```python
from build123d import *
from build123d import SkipClean  # not in build123d's __all__

# Parameters (mm, degrees)
F0_R     = 0.4
F1_DEPTH = 1.4
F2_DEPTH = 2.3
F3_DEPTH = 0.5


with BuildPart() as f1:
    # F0 (on Top) → F1 (new body)
    with BuildSketch(Plane.XY):
        with BuildLine():
            ThreePointArc((-2.7, 2.1476731595), (-1.1374313166, -3.2571076126), (3.45, 0))
            ThreePointArc((3.45, 0), (3.2571076126, 1.1374313166), (2.7, 2.1476731595))
            Line((2.7, 2.1476731595), (1.0139649895, 2.1476731595))
            ThreePointArc((1.0139649895, 2.1476731595), (2.0060897101, 1.2713099838), (2.375, 0))
            ThreePointArc((2.375, 0), (-1.2713099838, -2.0060897101), (-1.0139649895, 2.1476731595))
            Line((-1.0139649895, 2.1476731595), (-2.7, 2.1476731595))
        make_face()
        with BuildLine():
            Line((1.0139649895, 2.1476731595), (2.7, 2.1476731595))
            ThreePointArc((2.7, 2.1476731595), (0, 3.45), (-2.7, 2.1476731595))
            Line((-2.7, 2.1476731595), (-1.0139649895, 2.1476731595))
            ThreePointArc((-1.0139649895, 2.1476731595), (0, 2.375), (1.0139649895, 2.1476731595))
        make_face()
        with BuildLine():
            ThreePointArc((-2.7, 2.1476731595), (0, 3.45), (2.7, 2.1476731595))
            Line((2.7, 2.1476731595), (2.0471920173, 14.6072606371))
            ThreePointArc((2.0471920173, 14.6072606371), (2.0492978841, 14.553648693), (2.05, 14.5))
            ThreePointArc((2.05, 14.5), (-0.053648693, 12.4507021159), (-2.0471920173, 14.6072606371))
            Line((-2.0471920173, 14.6072606371), (-2.7, 2.1476731595))
        make_face()
        with BuildLine():
            ThreePointArc((2.05, 14.5), (2.0492978841, 14.553648693), (2.0471920173, 14.6072606371))
            ThreePointArc((2.0471920173, 14.6072606371), (0, 16.55), (-2.0471920173, 14.6072606371))
            ThreePointArc((-2.0471920173, 14.6072606371), (-0.053648693, 12.4507021159), (2.05, 14.5))
        make_face()
        with Locations((0, 14.5)):
            Circle(F0_R, mode=Mode.SUBTRACT)
    extrude(amount=F1_DEPTH)

    # F0 (on Top) → F2 (join)
    with BuildSketch(Plane.XY):
        with BuildLine():
            Line((1.0139649895, 2.1476731595), (2.7, 2.1476731595))
            ThreePointArc((2.7, 2.1476731595), (0, 3.45), (-2.7, 2.1476731595))
            Line((-2.7, 2.1476731595), (-1.0139649895, 2.1476731595))
            ThreePointArc((-1.0139649895, 2.1476731595), (0, 2.375), (1.0139649895, 2.1476731595))
        make_face()
        with BuildLine():
            ThreePointArc((-2.7, 2.1476731595), (-1.1374313166, -3.2571076126), (3.45, 0))
            ThreePointArc((3.45, 0), (3.2571076126, 1.1374313166), (2.7, 2.1476731595))
            Line((2.7, 2.1476731595), (1.0139649895, 2.1476731595))
            ThreePointArc((1.0139649895, 2.1476731595), (2.0060897101, 1.2713099838), (2.375, 0))
            ThreePointArc((2.375, 0), (-1.2713099838, -2.0060897101), (-1.0139649895, 2.1476731595))
            Line((-1.0139649895, 2.1476731595), (-2.7, 2.1476731595))
        make_face()
    with SkipClean():  # cleaning this boolean's faces spoils the solid; the shape is the same uncleaned
        extrude(amount=-F2_DEPTH)

    # F0 (on Top) → F3 (join)
    with BuildSketch(Plane.XY):
        with BuildLine():
            Line((0, 2.1476731595), (1.0139649895, 2.1476731595))
            ThreePointArc((1.0139649895, 2.1476731595), (0, 2.375), (-1.0139649895, 2.1476731595))
            Line((-1.0139649895, 2.1476731595), (0, 2.1476731595))
        make_face()
        with BuildLine():
            ThreePointArc((2.375, 0), (2.0060897101, 1.2713099838), (1.0139649895, 2.1476731595))
            Line((1.0139649895, 2.1476731595), (0, 2.1476731595))
            Line((0, 2.1476731595), (-1.0139649895, 2.1476731595))
            ThreePointArc((-1.0139649895, 2.1476731595), (-1.2713099838, -2.0060897101), (2.375, 0))
        make_face()
        with BuildLine():
            ThreePointArc((1.175, 0), (-0.8308504679, -0.8308504679), (0, 1.175))
            ThreePointArc((0, 1.175), (0.8308504679, 0.8308504679), (1.175, 0))
        make_face(mode=Mode.SUBTRACT)
    extrude(amount=F3_DEPTH)


solid = f1.part
```
Can you work these out from the model? Positions are in its coordinate system, mm. A direction names the side the tool comes from. Give positions to 0.01 mm unless a question says otherwise; leave off trailing zeros. Order: outer loops, then holes, each group sorted by start corner. A loop starts at its lowest first (then second) coordinate and runs counter-clockwise, first axis right, second up. Notation, with made-up numbers: (88.5, -26) - (118.5, -26) arc R29 ccw to (118.5, 2) - close; hole circle Ø4 at (-22.5, 9.25). An arc over 180 degrees is marked (long way). Use a Markdown table: item, result. Add a question column.
Q1. Please list where these lines run through material, in increasing order: line 1 along X through (y, z) = (0, 0.4) (3 decimals); line 2 along Z through (x, y) = (-1.5, 4.5); line 3 along Y through (x, z) = (1, 0.9).
Q2. If we mould it in two halves opening along X, with no side actions, what happens to faces 3 (the flat face through (-2.37, 8.46, 0.69)), 4 (the flat face through (0, 9, 0)), 5 (the flat face through (-1, 1, 0.5)), 6 (the flat face through (2.38, 8.29, 0.69))? For each: released by +X, released by -X, zero draft, split by the parting line, or undercut.
Q3. If we section it at C-C on z = -0.8: Write out the boundary of the cut face in (x, y) (3 decimals).
Q4. If we section it at D-D on x = 1.5: Write out the boundary of the cut face in (y, z), plus the area to 3 significant figures.
Q5. If we section it at B-B on y = -0.25: Write out the boundary of the cut face in (x, z).
Q6. On a 3-axis mill with a long thin cutter (end or side, diameter ignored), from which of +Z, -Z, +X, -X, +Y, -Y can I reach the whole of each face in a straight line? I mean faces 1 (the flat face through (-1, 1, 0)), 2 (the flat face through (0, 7, 1.4)). Say none if no direction works.
Q7. If we section it at A-A on z = 1.15: Write out the boundary of the cut face in (x, y) (3 decimals), plus the area to 3 significant figures.
Answers follow:
| question | item | result |
|---|---|---|
| 1 | line 1 | x = -3.45 to -1.175, 1.175 to 3.45 |
| 1 | line 2 | z = 0 to 1.4 |
| 1 | line 3 | y = -3.3 to -2.15, 2.15 to 16.29 |
| 2 | face 3 | released by -X |
| 2 | face 4 | zero draft |
| 2 | face 5 | undercut |
| 2 | face 6 | released by +X |
| 3 | outline | circle Ø6.9 at (0, 0); hole circle Ø4.75 at (0, 0) |
| 4 | outline | (-3.11, -2.3) - (-1.84, -2.3) - (-1.84, 0) - (1.84, 0) - (1.84, -2.3) - (3.11, -2.3) - (3.11, 0) - (15.9, 0) - (15.9, 1.4) - (1.84, 1.4) - (1.84, 0.5) - (-1.84, 0.5) - (-1.84, 1.4) - (-3.11, 1.4) - close |
| 4 | area | 29.1 mm^2 |
| 5 | outline | (-3.44, -2.3) - (-2.36, -2.3) - (-2.36, 0) - (-1.15, 0) - (-1.15, 0.5) - (-2.36, 0.5) - (-2.36, 1.4) - (-3.44, 1.4) - close; (1.15, 0) - (2.36, 0) - (2.36, -2.3) - (3.44, -2.3) - (3.44, 1.4) - (2.36, 1.4) - (2.36, 0.5) - (1.15, 0.5) - close |
| 6 | face 1 | -Z |
| 6 | face 2 | +Z, +X, -X, +Y, -Y |
| 7 | outline | (-2.7, 2.148) arc R3.45 ccw (long way) to (2.7, 2.148) - (2.047, 14.607) arc R2.05 ccw to (-2.047, 14.607) - close; hole circle Ø4.75 at (0, 0); hole circle Ø0.8 at (0, 14.5) |
| 7 | area | 79.6 mm^2 |
